Design review of the part built by this model. Coordinates are the model's own, in mm. A direction names the side the tool comes from. Give positions to 0.01 mm unless a question says otherwise; leave off trailing zeros. Write each loop counter-clockwise with the first axis right and the second up, starting at its lowest first coordinate (ties: lowest second). Pieces come first, ordered by that corner, then holes. Notation, with made-up numbers: (54.5, 3.25) -> (59.5, 3.25) arc R32 cw to (59.5, 34.25) -> close; hole circle Ø7 at (50, 31.25). An arc over 180 degrees is marked (long way). Put each result on its own line as item: value. Start each with the question number.
from build123d import *

# Parameters (mm, degrees)
F1_ANGLE_BACK = 59.9796203852
F1_ANGLE      = 119.9592407703


with BuildPart() as f1:
    # F0 (on Top) → F1 (revolve)
    with BuildSketch(Plane.XY, mode=Mode.PRIVATE) as f1_sk:
        Polygon((0, 183.6575716734), (0, 0), (77.6938870549, 0), (78.9715871215, 53.645722568), (144.7227597237, 51.4108687639), (151.7917811871, 0), (209.2998325825, 0), (195.5198347569, 59.4546198845), (109.4474121928, 176.6495704651), align=None)
    revolve(f1_sk.sketch.rotate(Axis((0, 91.8287858367, 0), (0, 1, 0)), -F1_ANGLE_BACK), axis=Axis((0, 91.8287858367, 0), (0, 1, 0)), revolution_arc=F1_ANGLE)


solid = f1.part
Q1. Mouldability with a two-part tool opening along Z and no side actions: class faces 1 (the face through (78.333, 27.198, 1.148)), 2 (the face through (44, 0, -2)), 3 (the face through (39.99, 93.11, 69.21)) as +Z half, -Z half, draft (parallel to the pull), parting line (faces both ways), or undercut.
Q2. Take a section at C-C on y = 107. Give the boundary of the cut face in (x, z), then the cut area to 3 significant figures.
Q3. To check wall thickness, follow probe 1 along Z at (x, y) = (124, 18); probe 2 along X at (y, z) = (91, 120); probe 3 along Z at (x, y) = (30, 137). State the ranges of each line that lie inside material, in increasing order. Write a range as from..to.
Q4. Take a section at B-B on y = 127. Give the boundary of the cut face in (x, z).
Q5. Machinability: for faces 4 (the face through (39.99, 93.11, -69.21)), 5 (the face through (147.5, 31.1, 2.2)), which of the approach directions +Z, -Z, +X, -X, +Y, -Y give a long, thin tool a straight path to every point of the face, cutting with its end or side? Answer none if there is none.
Q6. For pin 1 (1.5 mm diameter, centred on y = 144, z = -26, fed in from -X); pin 2 (5 mm diameter, centred on y = 122.5, z = -2, fed in from +X); pin 3 (1.5 mm diameter, centred on y = 145, z = -15.5, fed in from -X), all flat-tipped, find the tip position at first contact; note any pin that passes through.
Q7. Take a section at A-A on y = 13.5. Give the boundary of the cut face in (x, z).
Result:
1. face 1: undercut
1. face 2: draft
1. face 3: +Z half
2. outline: (0, 0) -> (80.35, -139.06) arc R160.6 ccw to (80.35, 139.06) -> close
2. area: 27,000 mm^2
3. probe 1: z = -163.41..-83.18, 83.18..163.41
3. probe 2: x = 69.34..123.71
3. probe 3: z = -51.92..51.92
4. outline: (0, 0) -> (73, -126.34) arc R145.91 ccw to (73, 126.34) -> close
5. face 4: -Z, -X, +Y, -Y
5. face 5: -Y
6. pin 1: stops at x = 14.59
6. pin 2: stops at x = 151.04
6. pin 3: stops at x = 8.52
7. outline: (0, 0) -> (39.03, -67.55) arc R78.02 ccw to (39.03, 67.55) -> close; (75.01, -129.82) -> (103.15, -178.51) arc R206.17 ccw to (103.15, 178.51) -> (75.01, 129.82) arc R149.94 cw to start
